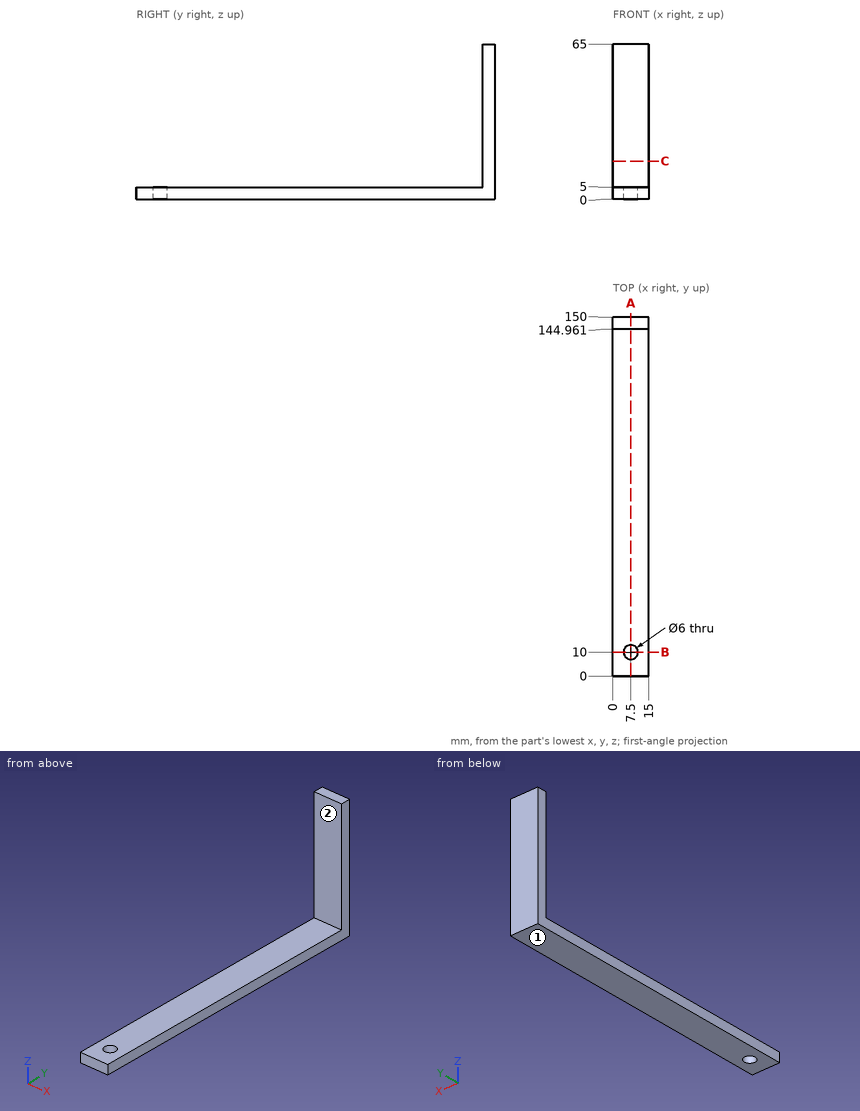
The figure shows three views and two pictorial views of one solid part (mm, origin at its lowest corner). Answer the questions. A direction names the side the tool comes from. Round coordinates to 2 decimals unless told otherwise and drop trailing zeros. Write each loop counter-clockwise with the first axis right and the second up, starting at its lowest first coordinate (ties: lowest second). Pieces come first, ordered by that corner, then holes. Notation, with made-up numbers: (0.5, -36) -> (43.5, -36) arc R29 ccw to (43.5, -1) -> close; hole circle Ø7 at (51.25, 56). An arc over 180 degrees is marked (long way). Answer as a JSON object with one key per item and string values. Group by question number.
Q1. Section C-C (z = 16) is taken. Write down the section's boundary in (x, y).
Q2. Straight lines are drawn through the part: line 1 along X through (y, z) = (10, 3.1); line 2 along Y through (x, z) = (7.5, 3.65); line 3 along Z through (x, y) = (13.25, 69). For each, find the intervals that lie inside material, in ascending order.
Q3. Each of these flat-tipped pins is pushed along its axis until it touches: pin 1 Ø1 at (x, z) = (6.5, 38) entering from -Y; pin 2 Ø7.5 at (x, y) = (10, 99) entering from +Z. Where does it stop, or does it pass through?
Q4. Section A-A (x = 7.5) is taken. Write down the section's boundary in (y, z), plus the area to 3 significant figures.
Q5. Which of the six approach directions +Z, -Z, +X, -X, +Y, -Y give full straight-line access (tool end or side, diameter ignored) to the marked faces 1 and 2?
Q6. Section B-B (y = 10) is taken. Write down the section's boundary in (x, z).
Check values:
{
 "1": {"outline": "(0, 144.96) -> (15, 144.96) -> (15, 150) -> (0, 150) -> close"},
 "2": {"line 1": "0 to 4.5, 10.5 to 15", "line 2": "0 to 7, 13 to 150", "line 3": "0 to 5"},
 "3": {"pin 1": "y = 144.96", "pin 2": "z = 5"},
 "4": {"outline": "(0, 0) -> (7, 0) -> (7, 5) -> (0, 5) -> close; (13, 0) -> (150, 0) -> (150, 65) -> (144.96, 65) -> (144.96, 5) -> (13, 5) -> close", "area": "1,020 mm^2"},
 "5": {"face 1": "-Z, +X, -X, +Y, -Y", "face 2": "+Z, +X, -X, -Y"},
 "6": {"outline": "(0, 0) -> (4.5, 0) -> (4.5, 5) -> (0, 5) -> close; (10.5, 0) -> (15, 0) -> (15, 5) -> (10.5, 5) -> close"}
}
